```python
from build123d import *

# Parameters (mm, degrees)
SKETCH_1_W          = 220
SKETCH_1_H          = 220
SKETCH_1_R          = 2.25
EXTRUDE_1_DEPTH     = 3
CUT_EXTRUDE_1_DEPTH = 156.592416268
FILLET_1_R          = 10
FILLET_START        = -1
FILLET_2_DEPTH      = 5
FILLET_2_2_DEPTH    = 3
SKETCH_4_R          = 1.75
CUT_EXTRUDE_2_DEPTH = 156.592416268
SKETCH1_R           = 15
CUT_EXTRUDE1_DEPTH  = 156.592416268


with BuildPart() as part:
    # Эскиз1 → Бобышка-Вытянуть1 (new body)
    with BuildSketch(Plane(origin=(0, 0, 0), x_dir=(1, 0, 0), z_dir=(0, 1, 0))):
        Rectangle(SKETCH_1_W, SKETCH_1_H)
        with Locations(Location((-20, 70, 0), (0, 0, 270))):
            Circle(SKETCH_1_R, mode=Mode.SUBTRACT)
        with Locations(Location((20, 70, 0), (0, 0, 90))):
            Circle(SKETCH_1_R, mode=Mode.SUBTRACT)
        with Locations(Location((-20, -80, 0), (0, 0, 90))):
            Circle(SKETCH_1_R, mode=Mode.SUBTRACT)
        with Locations(Location((20, -80, 0), (0, 0, 270))):
            Circle(SKETCH_1_R, mode=Mode.SUBTRACT)
        with Locations(Location((58.938080589, 42.735262449, 0), (0, 0, 270))):
            Circle(SKETCH_1_R, mode=Mode.SUBTRACT)
        with Locations(Location((72.618886322, 5.147557617, 0), (0, 0, 90))):
            Circle(SKETCH_1_R, mode=Mode.SUBTRACT)
        with Locations(Location((-72.618886322, 5.147557617, 0), (0, 0, 270))):
            Circle(SKETCH_1_R, mode=Mode.SUBTRACT)
        with Locations(Location((-58.938080589, 42.735262449, 0), (0, 0, 90))):
            Circle(SKETCH_1_R, mode=Mode.SUBTRACT)
    extrude(amount=EXTRUDE_1_DEPTH)

    # Эскиз3 → Вырез-Вытянуть1 (cut, through all)
    with BuildSketch(Plane(origin=(0, 3, 0), x_dir=(1, 0, 0), z_dir=(0, 1, 0))):
        Polygon((-110, 110), (-62, 110), (-62, 100), (-100, 100), (-100, 62), (-110, 62), align=None)
        Polygon((110, 62), (110, 110), (62, 110), (62, 100), (100, 100), (100, 62), align=None)
        Polygon((110, -110), (62, -110), (62, -100), (100, -100), (100, -62), (110, -62), align=None)
        Polygon((-110, -62), (-110, -110), (-62, -110), (-62, -100), (-100, -100), (-100, -62), align=None)
    extrude(amount=-CUT_EXTRUDE_1_DEPTH, mode=Mode.SUBTRACT)

    # Скругление1
    fillet_1_edges = [part.edges().sort_by_distance(p)[0] for p in [
        (-100, 1.5, 100),
        (100, 1.5, 100),
        (100, 1.5, -100),
        (-100, 1.5, -100),
    ]]
    fillet(fillet_1_edges, radius=FILLET_1_R)

    # Скругление2: read off the stored shape, not the designer's step
    # Скругление2 outline → Скругление2 (cut)
    with BuildSketch(Plane(origin=(0, 0, 0), x_dir=(1, 0, 0), z_dir=(0, 1, 0)).offset(FILLET_START)):
        with BuildLine():
            ThreePointArc((-105, -62), (-108.535533906, -60.535533906), (-110, -57))
            Line((-110, -57), (-110, -62))
            Line((-110, -62), (-105, -62))
        make_face()
        with BuildLine():
            ThreePointArc((-110, 57), (-108.535533906, 60.535533906), (-105, 62))
            Line((-105, 62), (-110, 62))
            Line((-110, 62), (-110, 57))
        make_face()
        with BuildLine():
            Line((62, 110), (57, 110))
            ThreePointArc((57, 110), (60.535533906, 108.535533906), (62, 105))
            Line((62, 105), (62, 110))
        make_face()
        with BuildLine():
            ThreePointArc((-62, 105), (-60.535533906, 108.535533906), (-57, 110))
            Line((-57, 110), (-62, 110))
            Line((-62, 110), (-62, 105))
        make_face()
        with BuildLine():
            ThreePointArc((62, -105), (60.535533906, -108.535533906), (57, -110))
            Line((57, -110), (62, -110))
            Line((62, -110), (62, -105))
        make_face()
        with BuildLine():
            ThreePointArc((-57, -110), (-60.535533906, -108.535533906), (-62, -105))
            Line((-62, -105), (-62, -110))
            Line((-62, -110), (-57, -110))
        make_face()
        with BuildLine():
            ThreePointArc((105, 62), (108.535533906, 60.535533906), (110, 57))
            Line((110, 57), (110, 62))
            Line((110, 62), (105, 62))
        make_face()
        with BuildLine():
            ThreePointArc((110, -57), (108.535533906, -60.535533906), (105, -62))
            Line((105, -62), (110, -62))
            Line((110, -62), (110, -57))
        make_face()
    extrude(amount=FILLET_2_DEPTH, mode=Mode.SUBTRACT)

    # Fillet 2 2 outline → Fillet 2 2 (add)
    with BuildSketch(Plane(origin=(0, 0, 0), x_dir=(1, 0, 0), z_dir=(0, 1, 0))):
        with BuildLine():
            Line((-100, 62), (-100, 67))
            ThreePointArc((-100, 67), (-101.464466094, 63.464466094), (-105, 62))
            Line((-105, 62), (-100, 62))
        make_face()
        with BuildLine():
            Line((-100, -62), (-105, -62))
            ThreePointArc((-105, -62), (-101.464466094, -63.464466094), (-100, -67))
            Line((-100, -67), (-100, -62))
        make_face()
        with BuildLine():
            Line((-62, 100), (-62, 105))
            ThreePointArc((-62, 105), (-63.464466094, 101.464466094), (-67, 100))
            Line((-67, 100), (-62, 100))
        make_face()
        with BuildLine():
            ThreePointArc((67, 100), (63.464466094, 101.464466094), (62, 105))
            Line((62, 105), (62, 100))
            Line((62, 100), (67, 100))
        make_face()
        with BuildLine():
            Line((62, -100), (62, -105))
            ThreePointArc((62, -105), (63.464466094, -101.464466094), (67, -100))
            Line((67, -100), (62, -100))
        make_face()
        with BuildLine():
            ThreePointArc((-67, -100), (-63.464466094, -101.464466094), (-62, -105))
            Line((-62, -105), (-62, -100))
            Line((-62, -100), (-67, -100))
        make_face()
        with BuildLine():
            Line((100, 62), (105, 62))
            ThreePointArc((105, 62), (101.464466094, 63.464466094), (100, 67))
            Line((100, 67), (100, 62))
        make_face()
        with BuildLine():
            ThreePointArc((100, -67), (101.464466094, -63.464466094), (105, -62))
            Line((105, -62), (100, -62))
            Line((100, -62), (100, -67))
        make_face()
    extrude(amount=FILLET_2_2_DEPTH)

    # Эскиз4 → Вырез-Вытянуть2 (cut, through all)
    with BuildSketch(Plane(origin=(0, 3, 0), x_dir=(1, 0, 0), z_dir=(0, 1, 0))):
        with Locations(Location((0, 105, 0), (0, 0, 270))):
            Circle(SKETCH_4_R)
        with Locations(Location((15, 105, 0), (0, 0, 270))):
            Circle(SKETCH_4_R)
        with Locations(Location((30, 105, 0), (0, 0, 270))):
            Circle(SKETCH_4_R)
        with Locations(Location((45, 105, 0), (0, 0, 270))):
            Circle(SKETCH_4_R)
        with Locations(Location((-15, 105, 0), (0, 0, 270))):
            Circle(SKETCH_4_R)
        with Locations(Location((-30, 105, 0), (0, 0, 270))):
            Circle(SKETCH_4_R)
        with Locations(Location((-45, 105, 0), (0, 0, 270))):
            Circle(SKETCH_4_R)
        with Locations(Location((105, 0, 0), (0, 0, 270))):
            Circle(SKETCH_4_R)
        with Locations(Location((105, -15, 0), (0, 0, 270))):
            Circle(SKETCH_4_R)
        with Locations(Location((105, -30, 0), (0, 0, 270))):
            Circle(SKETCH_4_R)
        with Locations(Location((105, -45, 0), (0, 0, 270))):
            Circle(SKETCH_4_R)
        with Locations(Location((105, 15, 0), (0, 0, 270))):
            Circle(SKETCH_4_R)
        with Locations(Location((105, 30, 0), (0, 0, 270))):
            Circle(SKETCH_4_R)
        with Locations(Location((105, 45, 0), (0, 0, 270))):
            Circle(SKETCH_4_R)
        with Locations(Location((0, -105, 0), (0, 0, 270))):
            Circle(SKETCH_4_R)
        with Locations(Location((-15, -105, 0), (0, 0, 270))):
            Circle(SKETCH_4_R)
        with Locations(Location((-30, -105, 0), (0, 0, 270))):
            Circle(SKETCH_4_R)
        with Locations(Location((-45, -105, 0), (0, 0, 270))):
            Circle(SKETCH_4_R)
        with Locations(Location((15, -105, 0), (0, 0, 270))):
            Circle(SKETCH_4_R)
        with Locations(Location((30, -105, 0), (0, 0, 270))):
            Circle(SKETCH_4_R)
        with Locations(Location((45, -105, 0), (0, 0, 270))):
            Circle(SKETCH_4_R)
        with Locations(Location((-105, 0, 0), (0, 0, 270))):
            Circle(SKETCH_4_R)
        with Locations(Location((-105, 15, 0), (0, 0, 270))):
            Circle(SKETCH_4_R)
        with Locations(Location((-105, 30, 0), (0, 0, 270))):
            Circle(SKETCH_4_R)
        with Locations(Location((-105, 45, 0), (0, 0, 270))):
            Circle(SKETCH_4_R)
        with Locations(Location((-105, -15, 0), (0, 0, 270))):
            Circle(SKETCH_4_R)
        with Locations(Location((-105, -30, 0), (0, 0, 270))):
            Circle(SKETCH_4_R)
        with Locations(Location((-105, -45, 0), (0, 0, 270))):
            Circle(SKETCH_4_R)
    extrude(amount=-CUT_EXTRUDE_2_DEPTH, mode=Mode.SUBTRACT)

    # Sketch1 → Cut-Extrude1 (cut, through all)
    with BuildSketch(Plane(origin=(0, 3, 0), x_dir=(1, 0, 0), z_dir=(0, 1, 0))):
        with Locations(Location((0, -20, 0), (0, 0, 270))):
            Circle(SKETCH1_R)
    extrude(amount=-CUT_EXTRUDE1_DEPTH, mode=Mode.SUBTRACT)


solid = part.part
```
Here's how the part is built. I have some questions about the finished solid (model axes, mm). Give positions to 0.01 mm unless a question says otherwise; leave off trailing zeros. Write each loop counter-clockwise with the first axis right and the second up, starting at its lowest first coordinate (ties: lowest second). Pieces come first, ordered by that corner, then holes. Notation, with made-up numbers: M 27,77 L 59,77 A5 cw 59,83 Z; hole C 10.5,-9.5 d1. An arc over 180 degrees is marked long. Put each result on its own line as item: value. Start each with the question number.
Item 1: Thinking about a two-plate mould opening in X: for faces 1 (the cylindrical face through (96.99, 1.48, -97.15)), 2 (the cylindrical face through (0.66, 1.521, 5.015)), 3 (the flat face through (-2, 0, -2)), which applies, +X half, -X half, draft (parallel to the pull), parting line (faces both ways), or undercut?
Item 2: I need wall thicknesses on L1, parallel to X at y = 1.5, z = 0; L2, parallel to Z at x = 21.5, y = 2.45; L3, parallel to X at y = 1.95, z = -28.5. Which ranges of each line are inside material? Lowest first, please. Write a range as from..to.
Item 3: If we section it at B-B, the plane x = 80.5: Write out the boundary of the cut face in (y, z), then the cut area to 3 significant figures.
Item 4: Will this pin go through, and if not, where does the flat tip stop? pin 1 (1.5 mm diameter, centred on x = -73.5, y = 1, fed in from +Z).
Item 5: If we section it at C-C, the plane y = 0.65: Count the separate pieces of the cut face and the enclosed holes in it, then the cut area to 3 significant figures.
Item 6: If we section it at A-A, the plane z = 20: Write out the boundary of the cut face in (x, y).
Values:
1. face 1: +X half
1. face 2: undercut
1. face 3: draft
2. L1: -110..-106.75, -103.25..103.25, 106.75..110
2. L2: -110..-71.68, -68.32..78.32, 81.68..110
2. L3: -110..-105.9, -104.1..104.1, 105.9..110
3. outline: M 0,-100 L 3,-100 L 3,100 L 0,100 Z
3. area: 600 mm²
4. pin 1: z = 100
5. separate pieces: 1
5. enclosed holes: 37
5. area: 43,800 mm²
6. outline: M -110,0 L -15,0 L -15,3 L -110,3 Z; M 15,0 L 110,0 L 110,3 L 15,3 Z
